Source: three-view drawing plus pictorial views. Frame: mm from the lowest corner of the part. A direction names the side the tool comes from. Give positions to 0.01 mm unless a question says otherwise; leave off trailing zeros. Loops run counter-clockwise (first coordinate to the right, second up) from the corner with the lowest first, then second, coordinate; pieces in that order, holes last.
1. Material intervals for line 1 along X through (y, z) = (7, 13.5); line 2 along Z through (x, y) = (29.5, 10), sorted ascending.
2. First-contact query: P1, Ø3, axis at x = 36.5, y = 7.5, coming from the +Z side; P2, Ø6, axis at x = 54, z = 3, coming from the -Y side; P3, Ø6, axis at x = 31, y = 12, coming from the -Z side. Flat tips, straight axial feed; report the tip coordinate or a pass-through.
3. Access query for the marked faces 1, 2 and 3. Directions: +Z, -Z, +X, -X, +Y, -Y. A direction counts if a zero-diameter tool reaches every point of the face in a straight line with its end or side. Return the directions, or none.
4. Section B-B, the plane z = 4. Output: boundary loops of the cut face in (x, y).
5. Section A-A, the plane x = 48. Output: boundary loops of the cut face in (y, z).
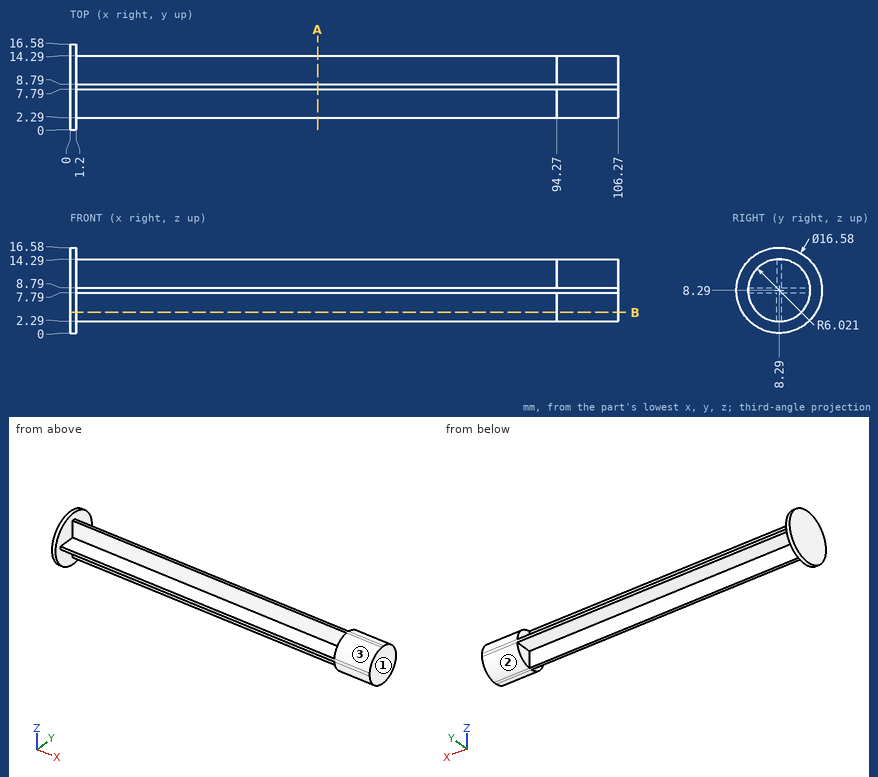
Answers below:
1. line 1: x = 0 to 1.2, 94.27 to 106.27
1. line 2: z = 7.79 to 8.79
2. P1: stops at z = 14.29
2. P2: stops at y = 7.79
2. P3: stops at z = 7.79
3. face 1: +Z, -Z, +X, +Y, -Y
3. face 2: -Z, +X, +Y
3. face 3: +Z, +X, -Y
4. outline: (0, 1.2) - (1.2, 1.2) - (1.2, 7.79) - (94.27, 7.79) - (94.27, 4.07) - (106.27, 4.07) - (106.27, 12.51) - (94.27, 12.51) - (94.27, 8.79) - (1.2, 8.79) - (1.2, 15.38) - (0, 15.38) - close
5. outline: (2.29, 7.79) - (7.79, 7.79) - (7.79, 2.29) - (8.79, 2.29) - (8.79, 7.79) - (14.29, 7.79) - (14.29, 8.79) - (8.79, 8.79) - (8.79, 14.29) - (7.79, 14.29) - (7.79, 8.79) - (2.29, 8.79) - close
